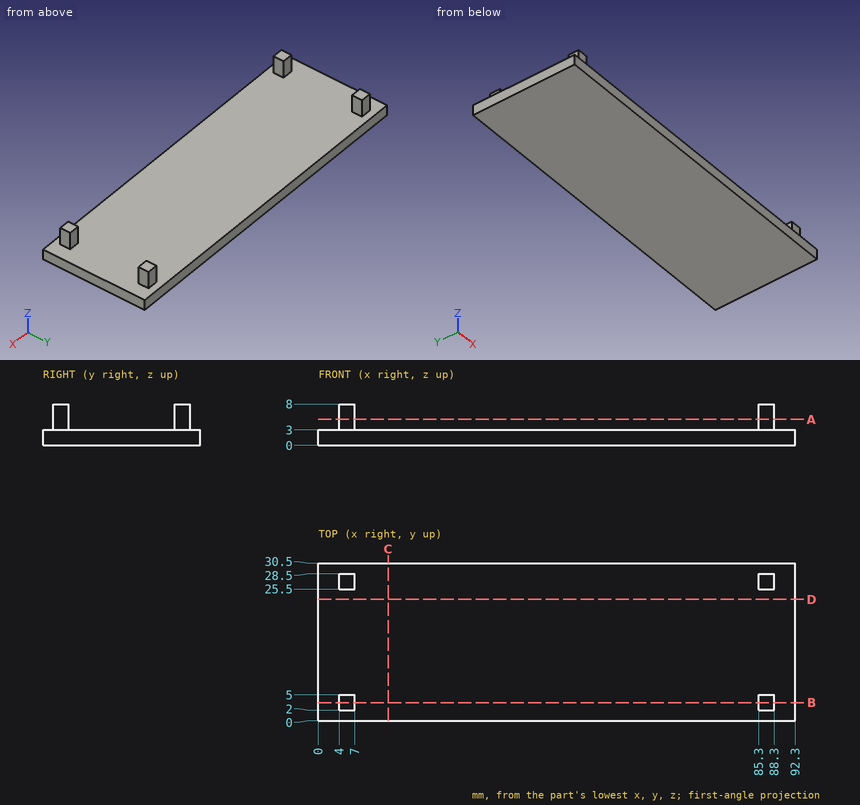
The figure shows three views and two pictorial views of one solid part (mm, origin at its lowest corner). Answer the questions. Coordinates: 2 decimals unless noted, no trailing zeros. Order: outer loops, then holes, each group sorted by start corner. A loop starts at its lowest first (then second) coordinate and runs counter-clockwise, first axis right, second up.
Q1. Consider line 1 (Y direction, x = 86, z = 5.5); line 2 (Z direction, x = 8, y = 10); line 3 (X direction, y = 27, z = 7). Determine where each line is inside the solid, lowest interval first.
Q2. Given P1, Ø2.5, axis at y = 4, z = 5, coming from the +X side; P2, Ø3.5, axis at x = 5, z = 5.5, coming from the +Y side; P3, Ø12, axis at x = 30, y = 13, coming from the +Z side, each flat-ended and moving along its own axis, determine where each tip first touches the part or whether it passes through.
Q3. A cutting plane is placed at B-B, the plane y = 3.5. Write down the section's boundary in (x, z), and give its area (3 significant figures).
Q4. A cutting plane is placed at C-C, the plane x = 13.5. Write down the section's boundary in (y, z), and give its area (3 significant figures).
Q5. A cutting plane is placed at A-A, the plane z = 5. Write down the section's boundary in (x, y), and give its area (3 significant figures).
Q6. A cutting plane is placed at D-D, the plane y = 23.5. Write down the section's boundary in (x, z).
Answers follow:
1. line 1: y = 2 to 5, 25.5 to 28.5
1. line 2: z = 0 to 3
1. line 3: x = 4 to 7, 85.3 to 88.3
2. P1: stops at x = 88.3
2. P2: stops at y = 28.5
2. P3: stops at z = 3
3. outline: (0, 0) - (92.3, 0) - (92.3, 3) - (88.3, 3) - (88.3, 8) - (85.3, 8) - (85.3, 3) - (7, 3) - (7, 8) - (4, 8) - (4, 3) - (0, 3) - close
3. area: 307 mm2
4. outline: (0, 0) - (30.5, 0) - (30.5, 3) - (0, 3) - close
4. area: 91.5 mm2
5. outline: (4, 2) - (7, 2) - (7, 5) - (4, 5) - close; (4, 25.5) - (7, 25.5) - (7, 28.5) - (4, 28.5) - close; (85.3, 2) - (88.3, 2) - (88.3, 5) - (85.3, 5) - close; (85.3, 25.5) - (88.3, 25.5) - (88.3, 28.5) - (85.3, 28.5) - close
5. area: 36.0 mm2
6. outline: (0, 0) - (92.3, 0) - (92.3, 3) - (0, 3) - close
